from build123d import *

# Parameters (mm, degrees)
F0_R           = 3.175
F1_DEPTH       = 44.45
F4_D           = 2.7178
F4_DEPTH       = 14.2875
F4_TIP         = 0.8165094952
F4_ON_F2_D     = 2.7178
F4_ON_F2_DEPTH = 14.2875
F4_ON_F2_TIP   = 0.8165094952


with BuildPart() as f1:
    # F0 (on Right) → F1 (new body, symmetric)
    with BuildSketch(Plane.YZ):
        Circle(F0_R)
    extrude(amount=F1_DEPTH, both=True)

    # F4
    with Locations(Plane(origin=(-44.45, 0, 0), x_dir=(0, -1, 0), z_dir=(-1, 0, 0))):
        with Locations((0, 0)):
            Hole(F4_D / 2, depth=F4_DEPTH)
            with Locations((0, 0, -(F4_DEPTH + F4_TIP / 2))):  # 118° drill point
                Cone(0, F4_D / 2, F4_TIP, mode=Mode.SUBTRACT)

    # F4 on F2
    with Locations(Plane.YZ.offset(44.45)):
        with Locations((0, 0)):
            Hole(F4_ON_F2_D / 2, depth=F4_ON_F2_DEPTH)
            with Locations((0, 0, -(F4_ON_F2_DEPTH + F4_ON_F2_TIP / 2))):  # 118° drill point
                Cone(0, F4_ON_F2_D / 2, F4_ON_F2_TIP, mode=Mode.SUBTRACT)


solid = f1.part
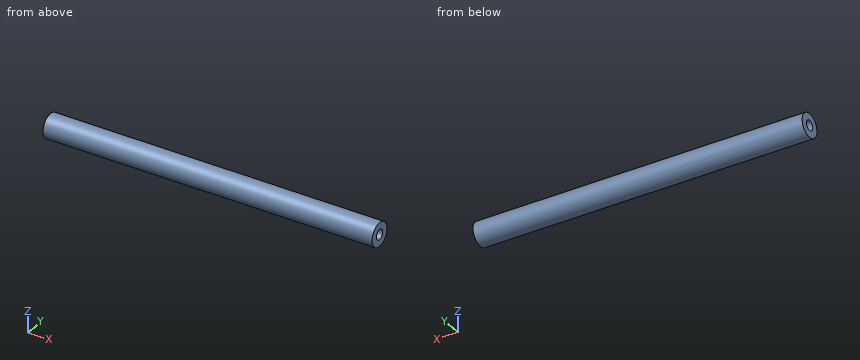
The model under review builds one solid part; all positions refer to its coordinate system, in mm. Give positions to 0.01 mm unless a question says otherwise; leave off trailing zeros. Loops run counter-clockwise (first coordinate to the right, second up) from the corner with the lowest first, then second, coordinate; pieces in that order, holes last. Notation, with made-up numbers: (39.5, 77.25) -> (46.5, 77.25) arc R22 ccw to (46.5, 86.25) -> close; hole circle Ø6 at (-30, 40). An arc over 180 degrees is marked (long way). Write each question's results on one line, items separated by ' | '.
1) For line 1 along Z through (x, y) = (39, 0) (3 decimals); line 2 along Y through (x, z) = (-37, 2.5); line 3 along Z through (x, y) = (40, -2), list the stretches that pass through material, from the lowest coordinate up. Write a range as from..to.
Conclusion:
line 1: z = -3.175..-1.359, 1.359..3.175 | line 2: y = -1.96..1.96 | line 3: z = -2.47..2.47
2) Take a section at A-A, the plane x = -10.5. Give the boundary of the cut face in (y, z) (3 decimals), plus the area to 3 significant figures.
Conclusion:
outline: circle Ø6.35 at (0, 0) | area: 31.7 mm^2
3) Insertion check: pin 1 Ø2 at (y, z) = (0, 0) entering from +X. The pin has a flat end and moves straight along its axis. Give the tip position at first contact, or say it passes through.
Conclusion:
pin 1: stops at x = 29.95
4) Take a section at B-B, the plane y = -2.25. Give the boundary of the cut face in (x, z).
Conclusion:
outline: (-44.45, -2.24) -> (44.45, -2.24) -> (44.45, 2.24) -> (-44.45, 2.24) -> close
